Can you work these out from the drawing? Everything is in mm from the part's minimum corner. Coordinates: 2 decimals unless noted, no trailing zeros. Loops run counter-clockwise (first coordinate to the right, second up) from the corner with the lowest first, then second, coordinate; pieces in that order, holes last. Notation, with made-up numbers: M 68,87 L 116,87 A25 ccw 116,99 Z; hole C 53.5,47 d8. An arc over 180 degrees is marked long. Use CSV: the item, a comma, the result in double quotes. Start each with the question number.
Q1. If we section it at D-D (y = 1.7): State how many separate pieces and enclosed holes the cut face has.
Q2. If we section it at C-C (z = 52.5): Please give me the cut outline in (x, y).
Q3. If we section it at A-A (z = 33): Please give me the cut outline in (x, y).
Q4. Please list where these lines run through material, in increasing order: probe 1 along Z at (x, y) = (11, 1.05); probe 2 along X at (y, z) = (0.3, 36); probe 3 along Z at (x, y) = (46, 1.55). Write a range as [from, to].
Q5. For pin 1 Ø4.5 at (x, z) = (35.19, 52.04) entering from +Y, with a flat end and sliding along its axis, tell me the tip position at first contact or that it passes through.
Q6. If we section it at B-B (x = 69): Please give me the cut outline in (y, z).
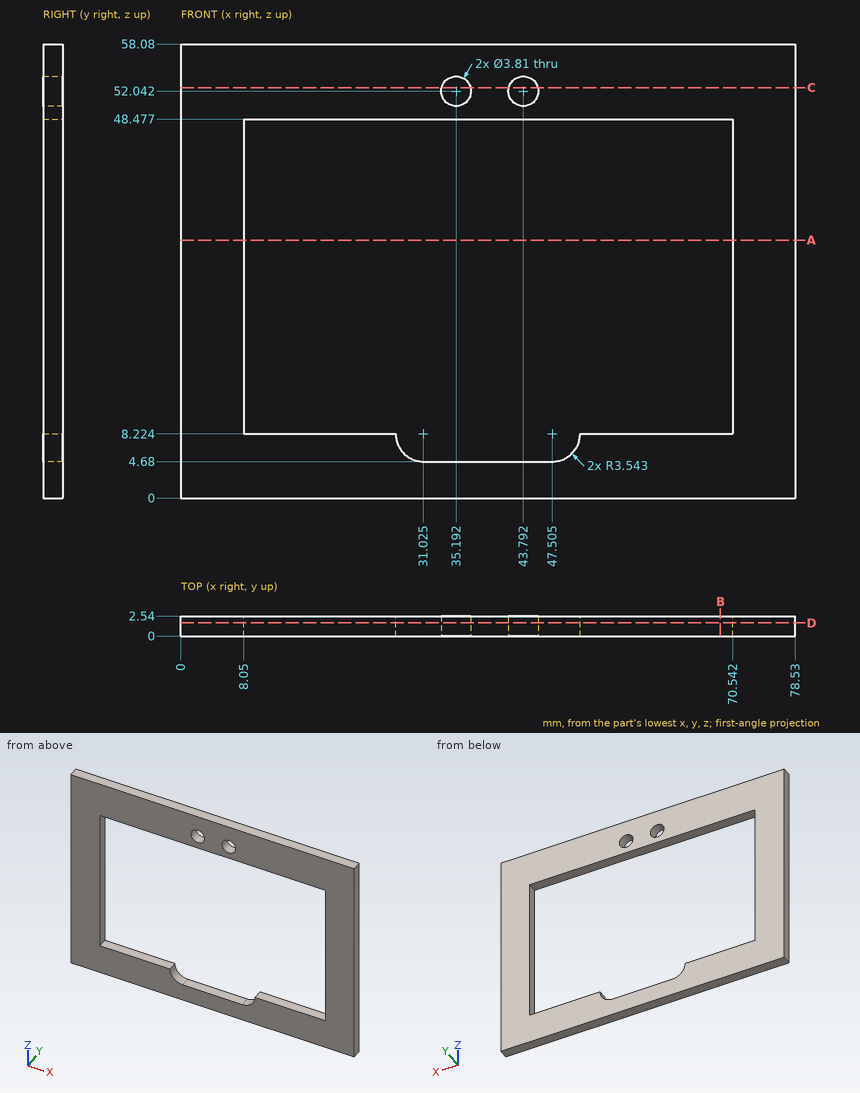
Results below:
1,separate pieces,"1"
1,enclosed holes,"3"
2,outline,"M 0,0 L 33.34,0 L 33.34,2.54 L 0,2.54 Z; M 37.04,0 L 41.94,0 L 41.94,2.54 L 37.04,2.54 Z; M 45.64,0 L 78.53,0 L 78.53,2.54 L 45.64,2.54 Z"
3,outline,"M 0,0 L 8.05,0 L 8.05,2.54 L 0,2.54 Z; M 70.54,0 L 78.53,0 L 78.53,2.54 L 70.54,2.54 Z"
4,probe 1,"[0, 8.22], [48.48, 58.08]"
4,probe 2,"[0, 8.05], [70.54, 78.53]"
4,probe 3,"[0, 4.68], [48.48, 58.08]"
5,pin 1,"y = 2.54"
6,outline,"M 0,0 L 2.54,0 L 2.54,8.22 L 0,8.22 Z; M 0,48.48 L 2.54,48.48 L 2.54,58.08 L 0,58.08 Z"
